from build123d import *

# Parameters (mm, degrees)
SCHIZZO1_R                   = 41
SCHIZZO1_R_2                 = 39
ESTRUSIONE_SOTTILE1_DEPTH    = 227.5
SCHIZZO2_R                   = 46
SCHIZZO2_R_2                 = 41
ESTRUSIONE_ESTRUSIONE1_DEPTH = 1
ESTRUSIONE_ESTRUSIONE2_START = -1
SCHIZZO3_R                   = 46
SCHIZZO3_R_2                 = 41
ESTRUSIONE_ESTRUSIONE2_DEPTH = 1


with BuildPart() as part:
    # Schizzo1 → Estrusione-Sottile1 (new, symmetric)
    with BuildSketch(Plane(origin=(0, 0, 0), x_dir=(1, 0, 0), z_dir=(0, 1, 0))):
        Circle(SCHIZZO1_R)
        Circle(SCHIZZO1_R_2, mode=Mode.SUBTRACT)
    extrude(amount=ESTRUSIONE_SOTTILE1_DEPTH, both=True)

    # Schizzo2 → Estrusione-Estrusione1 (add)
    with BuildSketch(Plane(origin=(0, 227.5, 0), x_dir=(1, 0, 0), z_dir=(0, 1, 0))):
        with Locations(Location((0, 0, 0), (0, 0, 270))):
            Circle(SCHIZZO2_R)
        with Locations(Location((0, 0, 0), (0, 0, 90))):
            Circle(SCHIZZO2_R_2, mode=Mode.SUBTRACT)
    extrude(amount=-ESTRUSIONE_ESTRUSIONE1_DEPTH)

    # Schizzo3 → Estrusione-Estrusione2 (add)
    with BuildSketch(Plane.XZ.offset(227.5).offset(ESTRUSIONE_ESTRUSIONE2_START)):
        with Locations(Location((0, 0, 0), (0, 0, 90))):
            Circle(SCHIZZO3_R)
        with Locations(Location((0, 0, 0), (0, 0, 270))):
            Circle(SCHIZZO3_R_2, mode=Mode.SUBTRACT)
    extrude(amount=ESTRUSIONE_ESTRUSIONE2_DEPTH)


solid = part.part
Verification items for the finished model (mm, model axes). A direction names the side the tool comes from. Coordinates: 2 decimals unless noted, no trailing zeros. Write each loop counter-clockwise with the first axis right and the second up, starting at its lowest first coordinate (ties: lowest second). Pieces come first, ordered by that corner, then holes. Notation, with made-up numbers: (-29.75, 12) -> (26.25, 12) arc R9 ccw to (26.25, 22) -> close; hole circle Ø4 at (-19.5, 77.5). An arc over 180 degrees is marked (long way). One line per item, written item: value. Start each with the question number.
Q1. Go/stop test with flat-tipped pins: P1, Ø2, axis at x = -22, y = 38.5, coming from the -Z side; P2, Ø1.5, axis at y = 127.5, z = -8.5, coming from the +X side; P3, Ø6, axis at x = -36, y = 45, coming from the +Z side. Record where each tip stops, or that it passes through.
Q2. Cross-section at B-B on z = 0. Enter the section's corners in (x, y), and give its area (3 significant figures).
Q3. Mould release check, pull along Y, two halves, no side actions. Record for faces 1 (the flat face through (10, 227.5, -38)), 2 (the cylindrical face through (-5.077, -3.185, -38.668)), 3 (the flat face through (3.2, -226.5, -41.1)): pulls with the +Y half, pulls with the -Y half, needs draft (parallel to the pull), parting line crosses it, or undercut.
Q4. Thickness scan on L1, parallel to Z at x = 0, y = -49; L2, parallel to Y at x = 25, z = 37.5; L3, parallel to X at y = -133.5, z = 15.5. Record the ranges inside material, lowest first. Write a range as from..to.
Q5. Cross-section at A-A on x = 0. Enter the section's corners in (y, z).
Q6. Access from +Z, -Z, +X, -X, +Y, -Y to the whole of each face (thin tool, end or side, straight path). Record for faces 4 (the flat face through (-3.2, 226.5, -41.1)), 5 (the cylindrical face through (38.787, 227.007, 24.729)).
Q7. Cross-section at C-C on y = 140. Enter the section's corners in (x, z).
Checked values:
1. P1: stops at z = -35.21
1. P2: stops at x = 40.26
1. P3: stops at z = 24.33
2. outline: (-46, -227.5) -> (-39, -227.5) -> (-39, 227.5) -> (-46, 227.5) -> (-46, 226.5) -> (-41, 226.5) -> (-41, -226.5) -> (-46, -226.5) -> close; (39, -227.5) -> (46, -227.5) -> (46, -226.5) -> (41, -226.5) -> (41, 226.5) -> (46, 226.5) -> (46, 227.5) -> (39, 227.5) -> close
2. area: 1,840 mm²
3. face 1: pulls with the +Y half
3. face 2: needs draft
3. face 3: undercut
4. L1: z = -41..-39, 39..41
4. L2: y = -227.5..-226.5, 226.5..227.5
4. L3: x = -37.96..-35.79, 35.79..37.96
5. outline: (-227.5, -46) -> (-226.5, -46) -> (-226.5, -41) -> (226.5, -41) -> (226.5, -46) -> (227.5, -46) -> (227.5, -39) -> (-227.5, -39) -> close; (-227.5, 39) -> (227.5, 39) -> (227.5, 46) -> (226.5, 46) -> (226.5, 41) -> (-226.5, 41) -> (-226.5, 46) -> (-227.5, 46) -> close
6. face 4: none
6. face 5: +Y, -Y
7. outline: circle Ø82 at (0, 0); hole circle Ø78 at (0, 0)
